```python
from build123d import *

# Parameters (mm, degrees)
F0_R     = 19.25
F1_DEPTH = 5
F2_R     = 16.75
F3_DEPTH = 2.5
F4_R     = 16.75
F5_DEPTH = 2.5
F6_SIZE  = 2.49999


# Not quite as in the source:
# - a fillet or chamfer is up to 0.001 mm smaller than in the source, because OpenCascade refuses the exact size


with BuildPart() as f1:
    # F0 (on Top) → F1 (new body)
    with BuildSketch(Plane.XY):
        Circle(F0_R)
    extrude(amount=F1_DEPTH)

    # F2 (on face) → F3 (join)
    with BuildSketch(Plane.XY.offset(5)):
        Circle(F2_R)
    extrude(amount=F3_DEPTH)

    # F4 (on face) → F5 (cut)
    with BuildSketch(Plane(origin=(0, 0, 0), x_dir=(1, 0, 0), z_dir=(0, 0, -1))):
        Circle(F4_R)
    extrude(amount=-F5_DEPTH, mode=Mode.SUBTRACT)

    # F6 (size 2.5 in the source; OpenCascade refuses exactly that, so slightly less here)
    f6_edges = [f1.edges().sort_by_distance(p)[0] for p in [
        (-19.25, 0, 5),
    ]]
    chamfer(f6_edges, length=F6_SIZE)


solid = f1.part
```
Here's how the part is built. I have some questions about the finished solid (model axes, mm). A direction names the side the tool comes from. Round coordinates to 2 decimals unless told otherwise and drop trailing zeros. Order: outer loops, then holes, each group sorted by start corner. A loop starts at its lowest first (then second) coordinate and runs counter-clockwise, first axis right, second up. Notation, with made-up numbers: M 79.5,31.5 L 90.5,31.5 A7 cw 90.5,35.5 Z; hole C -26.5,24 d8. An arc over 180 degrees is marked long. One line per question, with ' | ' between items.
1) For pin 1 Ø1.5 at (y, z) = (12.5, 3.5) entering from +X; pin 2 Ø6 at (x, y) = (-5, -1.5) entering from -Z; pin 3 Ø1 at (x, z) = (-11, 2) entering from +Y, each with a flat end and sliding along its axis, tell me the tip position at first contact or that it passes through.
Working result:
pin 1: x = 14.5 | pin 2: z = 2.5 | pin 3: y = 16.13
2) I need wall thicknesses on line 1 along Y through (x, z) = (0, 0.6); line 2 along X through (y, z) = (-0.5, 2); line 3 along Z through (x, y) = (7.5, -4). Which ranges of each line are inside material? Lowest first, please.
Working result:
line 1: -19.25 to -16.75, 16.75 to 19.25 | line 2: -19.24 to -16.74, 16.74 to 19.24 | line 3: 2.5 to 7.5
3) If we mould it in two halves opening along Y, with no side actions, what happens to faces 1 (the face through (0, 0, 7.5)), 2 (the face through (-15.28, -11.71, 1.23)), 3 (the face through (0, 0, 2.5)), 4 (the face through (-3.63, 16.35, 1.23))? For each: +Y half, -Y half, draft (parallel to the pull), parting line (faces both ways), or undercut.
Working result:
face 1: draft | face 2: parting line | face 3: undercut | face 4: undercut
4) I want a section at C-C, the plane z = 3.5. Write out the boundary of the cut face in (x, y), then the cut area to 3 significant figures.
Working result:
outline: C 0,0 d36.5 | area: 1,050 mm²
5) I want a section at D-D, the plane z = 1.25. Write out the boundary of the cut face in (x, y), then the cut area to 3 significant figures.
Working result:
outline: C 0,0 d38.5; hole C 0,0 d33.5 | area: 283 mm²
6) For faces 5 (the face through (-3.63, -16.35, 6.23)), 6 (the face through (-2, -17, 0)), which set-ups out of +Z, -Z, +X, -X, +Y, -Y let a thin tool reach every point of the face, with its end or its side?
Working result:
face 5: +Z | face 6: -Z, +X, -X, +Y, -Y
